The drawing under review shows one solid part. Ordinate dimensions are in mm from its lowest x, y, z. Coordinates: 2 decimals unless noted, no trailing zeros. Write each loop counter-clockwise with the first axis right and the second up, starting at its lowest first coordinate (ties: lowest second). Pieces come first, ordered by that corner, then holes.
1) Add section B-B, the plane x = 99.75. State the section outline as (y, z) points, then the cut area to 3 significant figures.
2) For line 1 (Y direction, x = 89.5, z = 1.4); line 2 (Y direction, x = 99.75, z = 0.6); line 3 (X direction, y = 14, z = 2.9), list the stretches that pass through material, from the lowest coordinate up.
3) Add section A-A, the plane y = 18. State the section outline as (x, z) points, then the cut area to 3 significant figures.
4) Add section C-C, the plane z = 0.9. State the section outline as (x, y) points.
5) Add section D-D, the plane y = 30.5. State the section outline as (x, z) points.
6) For P1, Ø0.8, axis at y = 18, z = 2, coming from the +X side; P2, Ø5.5, axis at x = 89.5, y = 18, coming from the -Z side; P3, Ø1.2, axis at x = 49, z = 2.5, coming from the +Y side, all flat-tipped, find the tip position at first contact; note any pin that passes through.
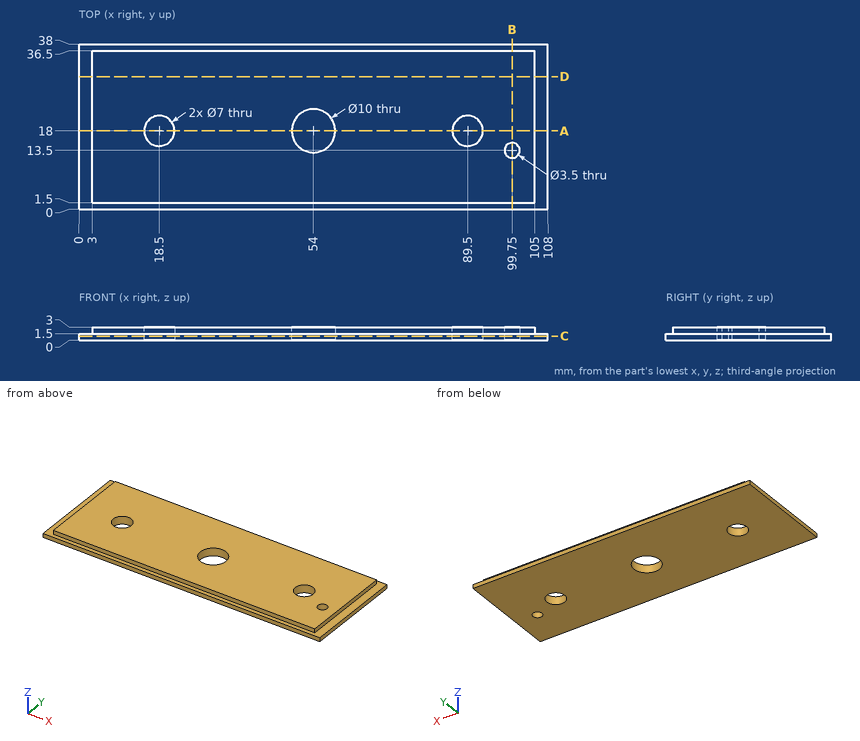
Geometry results:
1. outline: (0, 0) - (11.75, 0) - (11.75, 3) - (1.5, 3) - (1.5, 1.5) - (0, 1.5) - close; (15.25, 0) - (38, 0) - (38, 1.5) - (36.5, 1.5) - (36.5, 3) - (15.25, 3) - close
1. area: 99.0 mm2
2. line 1: y = 0 to 14.5, 21.5 to 38
2. line 2: y = 0 to 11.75, 15.25 to 38
2. line 3: x = 3 to 51, 57 to 98.07, 101.43 to 105
3. outline: (0, 0) - (15, 0) - (15, 3) - (3, 3) - (3, 1.5) - (0, 1.5) - close; (22, 0) - (49, 0) - (49, 3) - (22, 3) - close; (59, 0) - (86, 0) - (86, 3) - (59, 3) - close; (93, 0) - (108, 0) - (108, 1.5) - (105, 1.5) - (105, 3) - (93, 3) - close
3. area: 243 mm2
4. outline: (0, 0) - (108, 0) - (108, 38) - (0, 38) - close; hole circle Ø7 at (18.5, 18); hole circle Ø10 at (54, 18); hole circle Ø7 at (89.5, 18); hole circle Ø3.5 at (99.75, 13.5)
5. outline: (0, 0) - (108, 0) - (108, 1.5) - (105, 1.5) - (105, 3) - (3, 3) - (3, 1.5) - (0, 1.5) - close
6. P1: stops at x = 105
6. P2: passes through
6. P3: stops at y = 36.5
